Input: dimensioned drawing with shaded views. Units: mm. Origin: part minimum x, y, z. Round coordinates to 2 decimals unless told otherwise and drop trailing zeros. Loops run counter-clockwise (first coordinate to the right, second up) from the corner with the lowest first, then second, coordinate; pieces in that order, holes last.
1) Ray query, line 1 along Z through (x, y) = (45, 1.6); line 2 along X through (y, z) = (1.1, 31.5). Return the intervals inside material, ascending.
2) Section A-A, the plane x = 45. Return loops of the section in (y, z), and give its area (3 significant figures).
3) Section B-B, the plane z = 17.5. Return loops of the section in (x, y).
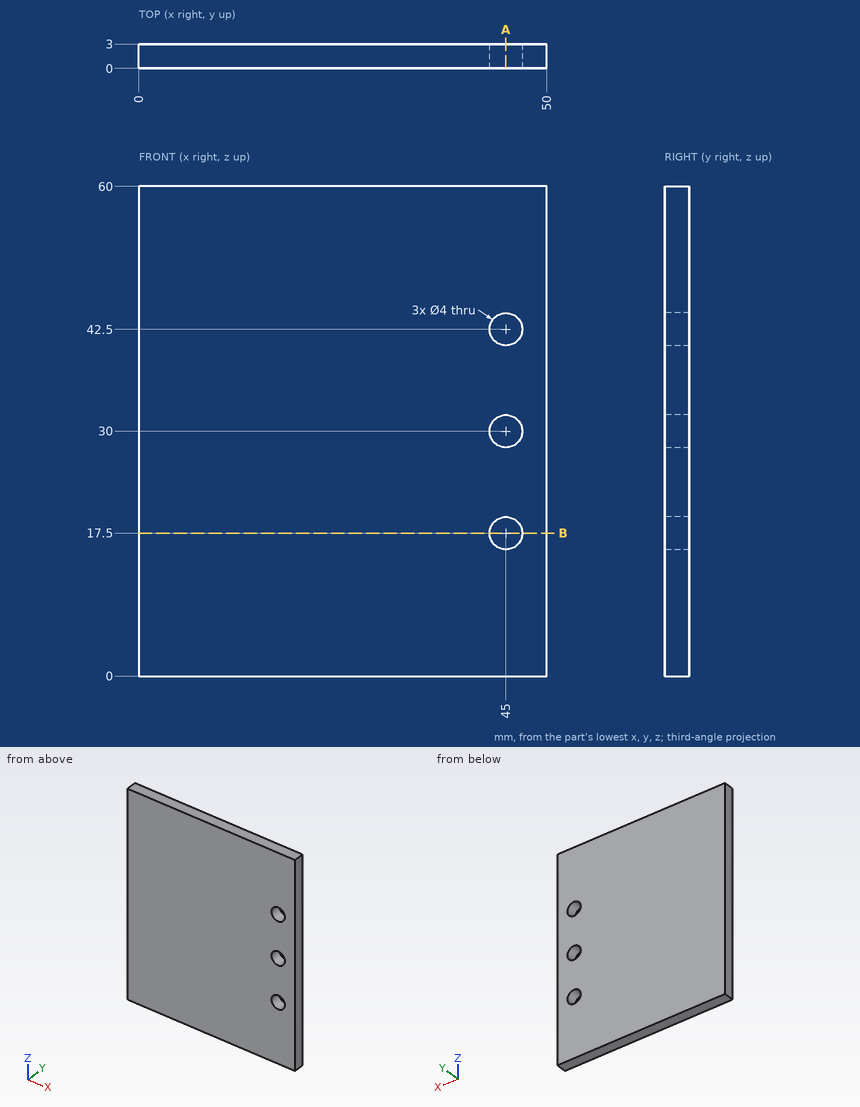
Final values:
1. line 1: z = 0 to 15.5, 19.5 to 28, 32 to 40.5, 44.5 to 60
1. line 2: x = 0 to 43.68, 46.32 to 50
2. outline: (0, 0) - (3, 0) - (3, 15.5) - (0, 15.5) - close; (0, 19.5) - (3, 19.5) - (3, 28) - (0, 28) - close; (0, 32) - (3, 32) - (3, 40.5) - (0, 40.5) - close; (0, 44.5) - (3, 44.5) - (3, 60) - (0, 60) - close
2. area: 144 mm2
3. outline: (0, 0) - (43, 0) - (43, 3) - (0, 3) - close; (47, 0) - (50, 0) - (50, 3) - (47, 3) - close
